from build123d import *

# Parameters (mm, degrees)
SKETCH_2_W          = 17.6
SKETCH_2_H          = 38.1
EXTRUDE_2_DEPTH     = 1
CUT_EXTRUDE_3_REACH = 23.008
SKETCH_3_W          = 7
SKETCH_3_H          = 2.5
SKETCH_3_W_2        = 3
SKETCH_3_H_2        = 3


with BuildPart() as part:
    # 草圖2 → 伸長2 (new body)
    with BuildSketch(Plane(origin=(0, 0, 0), x_dir=(1, 0, 0), z_dir=(0, 1, 0))):
        Rectangle(SKETCH_2_W, SKETCH_2_H)
    extrude(amount=EXTRUDE_2_DEPTH)

    # 草圖3 → 伸長3 (cut, up to next)
    with BuildSketch(Plane(origin=(0, 1, 0), x_dir=(1, 0, 0), z_dir=(0, 1, 0)), mode=Mode.PRIVATE) as cut_extrude_3_sk1:
        with Locations((0, 17.8)):
            Rectangle(SKETCH_3_W, SKETCH_3_H)
    cut_extrude_3_tool1 = extrude(cut_extrude_3_sk1.sketch, amount=-CUT_EXTRUDE_3_REACH, mode=Mode.PRIVATE) & part.part
    # 草圖3 → 伸長3 (cut, up to next)
    with BuildSketch(Plane(origin=(0, 1, 0), x_dir=(1, 0, 0), z_dir=(0, 1, 0)), mode=Mode.PRIVATE) as cut_extrude_3_sk2:
        with BuildLine():
            Line((8.8, 19.05), (6.3, 19.05))
            Line((6.3, 19.05), (6.3, 17.55))
            ThreePointArc((6.3, 17.55), (6.592893219, 16.842893219), (7.3, 16.55))
            Line((7.3, 16.55), (8.8, 16.55))
            Line((8.8, 16.55), (8.8, 19.05))
        make_face()
    cut_extrude_3_tool2 = extrude(cut_extrude_3_sk2.sketch, amount=-CUT_EXTRUDE_3_REACH, mode=Mode.PRIVATE) & part.part
    # 草圖3 → 伸長3 (cut, up to next)
    with BuildSketch(Plane(origin=(0, 1, 0), x_dir=(1, 0, 0), z_dir=(0, 1, 0)), mode=Mode.PRIVATE) as cut_extrude_3_sk3:
        with BuildLine():
            Line((-8.8, 19.05), (-6.3, 19.05))
            Line((-6.3, 19.05), (-6.3, 17.55))
            ThreePointArc((-6.3, 17.55), (-6.592893219, 16.842893219), (-7.3, 16.55))
            Line((-7.3, 16.55), (-8.8, 16.55))
            Line((-8.8, 16.55), (-8.8, 19.05))
        make_face()
    cut_extrude_3_tool3 = extrude(cut_extrude_3_sk3.sketch, amount=-CUT_EXTRUDE_3_REACH, mode=Mode.PRIVATE) & part.part
    # 草圖3 → 伸長3 (cut, up to next)
    with BuildSketch(Plane(origin=(0, 1, 0), x_dir=(1, 0, 0), z_dir=(0, 1, 0)), mode=Mode.PRIVATE) as cut_extrude_3_sk4:
        with BuildLine():
            Line((-8.8, -19.05), (-6.3, -19.05))
            Line((-6.3, -19.05), (-6.3, -17.55))
            ThreePointArc((-6.3, -17.55), (-6.592893219, -16.842893219), (-7.3, -16.55))
            Line((-7.3, -16.55), (-8.8, -16.55))
            Line((-8.8, -16.55), (-8.8, -19.05))
        make_face()
    cut_extrude_3_tool4 = extrude(cut_extrude_3_sk4.sketch, amount=-CUT_EXTRUDE_3_REACH, mode=Mode.PRIVATE) & part.part
    # 草圖3 → 伸長3 (cut, up to next)
    with BuildSketch(Plane(origin=(0, 1, 0), x_dir=(1, 0, 0), z_dir=(0, 1, 0)), mode=Mode.PRIVATE) as cut_extrude_3_sk5:
        with BuildLine():
            Line((7.3, -16.55), (8.8, -16.55))
            Line((8.8, -16.55), (8.8, -19.05))
            Line((8.8, -19.05), (6.3, -19.05))
            Line((6.3, -19.05), (6.3, -17.55))
            ThreePointArc((6.3, -17.55), (6.592893219, -16.842893219), (7.3, -16.55))
        make_face()
    cut_extrude_3_tool5 = extrude(cut_extrude_3_sk5.sketch, amount=-CUT_EXTRUDE_3_REACH, mode=Mode.PRIVATE) & part.part
    # 草圖3 → 伸長3 (cut, up to next)
    with BuildSketch(Plane(origin=(0, 1, 0), x_dir=(1, 0, 0), z_dir=(0, 1, 0)), mode=Mode.PRIVATE) as cut_extrude_3_sk6:
        with BuildLine():
            Line((-7.8, -9.55), (-2.598076211, -9.55))
            ThreePointArc((-2.598076211, -9.55), (3, -11.05), (-2.598076211, -12.55))
            Line((-2.598076211, -12.55), (-7.8, -12.55))
            Line((-7.8, -12.55), (-7.8, -9.55))
        make_face()
    cut_extrude_3_tool6 = extrude(cut_extrude_3_sk6.sketch, amount=-CUT_EXTRUDE_3_REACH, mode=Mode.PRIVATE) & part.part
    # 草圖3 → 伸長3 (cut, up to next)
    with BuildSketch(Plane(origin=(0, 1, 0), x_dir=(1, 0, 0), z_dir=(0, 1, 0)), mode=Mode.PRIVATE) as cut_extrude_3_sk7:
        with Locations((5.8, -11.05)):
            Rectangle(SKETCH_3_W_2, SKETCH_3_H_2)
    cut_extrude_3_tool7 = extrude(cut_extrude_3_sk7.sketch, amount=-CUT_EXTRUDE_3_REACH, mode=Mode.PRIVATE) & part.part
    add(cut_extrude_3_tool1.solids().sort_by_distance((0, 1, -17.8))[0], mode=Mode.SUBTRACT)
    add(cut_extrude_3_tool2.solids().sort_by_distance((7.586504, 1, -17.836504))[0], mode=Mode.SUBTRACT)
    add(cut_extrude_3_tool3.solids().sort_by_distance((-7.586504, 1, -17.836504))[0], mode=Mode.SUBTRACT)
    add(cut_extrude_3_tool4.solids().sort_by_distance((-7.586504, 1, 17.836504))[0], mode=Mode.SUBTRACT)
    add(cut_extrude_3_tool5.solids().sort_by_distance((7.586504, 1, 17.836504))[0], mode=Mode.SUBTRACT)
    add(cut_extrude_3_tool6.solids().sort_by_distance((-1.831773, 1, 11.05))[0], mode=Mode.SUBTRACT)
    add(cut_extrude_3_tool7.solids().sort_by_distance((5.8, 1, 11.05))[0], mode=Mode.SUBTRACT)


solid = part.part
Could you check a few things on this model? Use its own coordinates, in mm. A direction names the side the tool comes from. Round coordinates to 2 decimals unless told otherwise and drop trailing zeros. Write each loop counter-clockwise with the first axis right and the second up, starting at its lowest first coordinate (ties: lowest second). Pieces come first, ordered by that corner, then holes. Notation, with made-up numbers: (21.5, -12) -> (55.5, -12) arc R24 ccw to (55.5, 4) -> close; hole circle Ø1 at (41, 40). An arc over 180 degrees is marked (long way). Use a Markdown table: item, result.
1. If we section it at A-A (x = -5.75): List the corners of the cut face in (y, z) for me.
Answer key:
| item | result |
|---|---|
| outline | (0, -19.05) -> (1, -19.05) -> (1, 9.55) -> (0, 9.55) -> close; (0, 12.55) -> (1, 12.55) -> (1, 19.05) -> (0, 19.05) -> close |
2. If we section it at D-D (x = 0): List the corners of the cut face in (y, z) for me, then the cut area to 3 significant figures.
Answer key:
| item | result |
|---|---|
| outline | (0, -16.55) -> (1, -16.55) -> (1, 8.05) -> (0, 8.05) -> close; (0, 14.05) -> (1, 14.05) -> (1, 19.05) -> (0, 19.05) -> close |
| area | 29.6 mm^2 |
3. If we section it at C-C (y = 0.75): List the corners of the cut face in (x, z) for me, then the cut area to 3 significant figures.
Answer key:
| item | result |
|---|---|
| outline | (-8.8, -16.55) -> (-7.3, -16.55) arc R1 cw to (-6.3, -17.55) -> (-6.3, -19.05) -> (-3.5, -19.05) -> (-3.5, -16.55) -> (3.5, -16.55) -> (3.5, -19.05) -> (6.3, -19.05) -> (6.3, -17.55) arc R1 cw to (7.3, -16.55) -> (8.8, -16.55) -> (8.8, 16.55) -> (7.3, 16.55) arc R1 cw to (6.3, 17.55) -> (6.3, 19.05) -> (-6.3, 19.05) -> (-6.3, 17.55) arc R1 cw to (-7.3, 16.55) -> (-8.8, 16.55) -> close; hole (-7.8, 9.55) -> (-2.6, 9.55) arc R3 ccw (long way) to (-2.6, 12.55) -> (-7.8, 12.55) -> close; hole (4.3, 9.55) -> (7.3, 9.55) -> (7.3, 12.55) -> (4.3, 12.55) -> close |
| area | 577 mm^2 |
4. Please list where these lines run through material, in increasing order: probe 1 along X at (y, z) = (0.2, 11); probe 2 along Z at (x, y) = (-5.25, 0.95); probe 3 along Z at (x, y) = (-7.5, 0.9).
Answer key:
| item | result |
|---|---|
| probe 1 | x = -8.8 to -7.8, 3 to 4.3, 7.3 to 8.8 |
| probe 2 | z = -19.05 to 9.55, 12.55 to 19.05 |
| probe 3 | z = -16.55 to 9.55, 12.55 to 16.55 |
5. If we section it at B-B (z = 11.05): List the corners of the cut face in (x, y) for me, then the cut area to 3 significant figures.
Answer key:
| item | result |
|---|---|
| outline | (-8.8, 0) -> (-7.8, 0) -> (-7.8, 1) -> (-8.8, 1) -> close; (3, 0) -> (4.3, 0) -> (4.3, 1) -> (3, 1) -> close; (7.3, 0) -> (8.8, 0) -> (8.8, 1) -> (7.3, 1) -> close |
| area | 3.80 mm^2 |
6. For pin 1 Ø0.5 at (x, y) = (-1.5, 0.5) entering from -Z, with a flat end and sliding along its axis, tell me the tip position at first contact or that it passes through.
Answer key:
| item | result |
|---|---|
| pin 1 | stops at z = -16.55 |
7. Which directions (+Z, -Z, +X, -X, +Y, -Y) give clear straight access to the entire face, cutting with the end or side of a thin tool? Please do faces 4 (the face through (8, 0.5, 16.55)), 5 (the face through (-3.5, 0.5, -17.8)), 6 (the face through (6.3, 0.5, -18.3)), 7 (the face through (-8, 0.5, -16.55)).
Answer key:
| item | result |
|---|---|
| face 4 | +Z, +X, +Y, -Y |
| face 5 | -Z, +Y, -Y |
| face 6 | -Z, +X, +Y, -Y |
| face 7 | -Z, -X, +Y, -Y |
8. We'd pull the mould along X, two halves only. Please class faces 1 (the face through (-0.1, 0.5, 19.05)), 2 (the face through (0, 0.5, -16.55)), 3 (the face through (8.8, 0.5, 0.2)): +X half, -X half, draft (parallel to the pull), parting line (faces both ways), or undercut.
Answer key:
| item | result |
|---|---|
| face 1 | draft |
| face 2 | undercut |
| face 3 | +X half |
